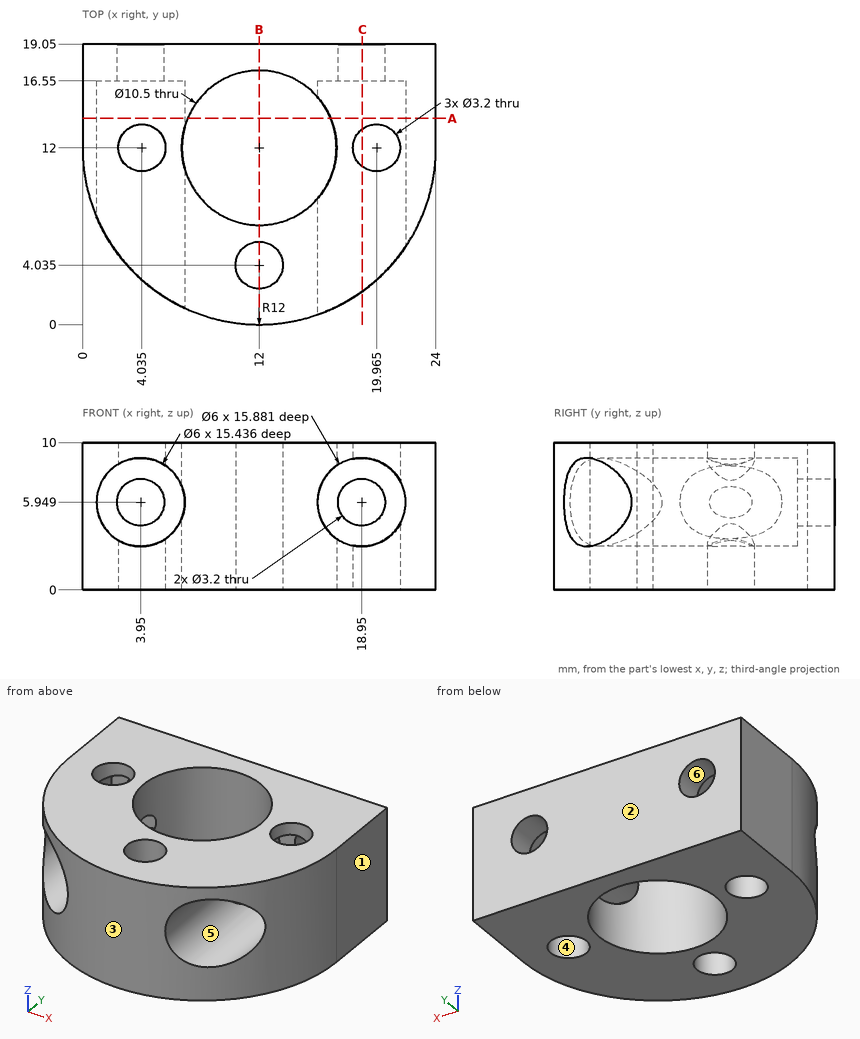
Geometry: see drawing. Coordinates: mm, zero at the bounding-box minimum. A direction names the side the tool comes from. Coordinates: 2 decimals unless noted, no trailing zeros. Order: outer loops, then holes, each group sorted by start corner. A loop starts at its lowest first (then second) coordinate and runs counter-clockwise, first axis right, second up. Notation, with made-up numbers: M -22,36.25 L -18,36.25 A18 ccw -18,62.25 Z; hole C 5,29 d5. An arc over 180 degrees is marked long. Write item = value, one per line. Start each with the question number.
(1) Pull-direction query (Y, two-part tool) for the marked faces 1, 2, 3 and 4; classes: released by +Y, released by -Y, zero draft, split by the parting line, or undercut.
(2) Section C-C on x = 19. Output: boundary loops of the cut face in (y, z).
(3) Section B-B on x = 12. Give the number of separate pieces and of enclosed holes in the cut face, and give its area (3 significant figures).
(4) Line query: line 1 along X through (y, z) = (10.5, 4.75) (1 decimal); line 2 along X through (y, z) = (16.5, 2) (1 decimal); line 3 along X through (y, z) = (9, 3.25) (1 decimal). Output: solid intervals per line, ascending. Write a range as [from, to].
(5) Section A-A on y = 14. Output: boundary loops of the cut face in (x, z).
(6) Reachability of the marked faces 5 and 6 from +Z, -Z, +X, -X, +Y, -Y: full face, straight path, thin tool, end or side. Return the list, or none.
(7) First-contact query: P1, Ø3.5, axis at x = 4.04, y = 12, coming from the +Z side; P2, Ø2, axis at y = 8, z = 7, coming from the -X side; P3, Ø5, axis at x = 3, z = 4.5, coming from the -Y side; P4, Ø3, axis at x = 3.95, z = 5.95, coming from the +Y side. Flat tips, straight axial feed; report the tip coordinate or a pass-through.
Result set:
q1.face_1 = zero draft
q1.face_2 = released by +Y
q1.face_3 = released by -Y
q1.face_4 = undercut
q2.outline = M 2.25,0 L 10.72,0 L 10.72,2.95 L 2.25,2.95 Z; M 2.25,8.95 L 10.72,8.95 L 10.72,10 L 2.25,10 Z; M 13.28,0 L 19.05,0 L 19.05,4.35 L 16.55,4.35 L 16.55,2.95 L 13.28,2.95 Z; M 13.28,8.95 L 16.55,8.95 L 16.55,7.55 L 19.05,7.55 L 19.05,10 L 13.28,10 Z
q3.separate_pieces = 3
q3.enclosed_holes = 0
q3.area = 53.5 mm²
q4.line_1 = [0.1, 1.2], [6.7, 7], [21.7, 23.9]
q4.line_2 = [0, 9.3], [14.7, 24]
q4.line_3 = [0.4, 2.6], [5.3, 7.7], [16.3, 17.6], [20.3, 23.6]
q5.outline = M 0,0 L 7.15,0 L 7.15,10 L 0,10 Z; M 16.85,0 L 24,0 L 24,10 L 16.85,10 L 16.85,8.1 A3 cw long 16.85,3.8 Z; hole C 3.95,5.95 d6
q6.face_5 = -Y
q6.face_6 = +Y, -Y
q7.P1 = 10
q7.P2 = 0.38
q7.P3 = 2.16
q7.P4 = through
